from build123d import *

# Parameters (mm, degrees)
F0_W     = 6.35
F0_H     = 28.575
F0_H_2   = 31.75
F0_W_2   = 69.723
F1_DEPTH = 25.4
F2_DEPTH = 6.35
F3_DEPTH = 6.35
F4_DEPTH = 11.176
F7_DEPTH = 6.35


with BuildPart() as f1:
    # F0 (on Top) → F1 (new body)
    with BuildSketch(Plane.XY):
        with Locations((3.175, 14.2875)):
            Rectangle(F0_W, F0_H)
        Polygon((6.35, 28.575), (6.35, 0), (69.596, 0), (69.596, 17.526), (87.122, 17.526), (76.073, 28.575), align=None)
        with BuildLine():
            ThreePointArc((30.988, 8.636), (25.4, 14.224), (30.988, 19.812))
            Line((30.988, 19.812), (54.864, 19.812))
            ThreePointArc((54.864, 19.812), (60.452, 14.224), (54.864, 8.636))
            Line((54.864, 8.636), (30.988, 8.636))
        make_face(mode=Mode.SUBTRACT)
        with Locations((3.175, 44.45)):
            Rectangle(F0_W, F0_H_2)
        Polygon((69.596, 17.526), (69.596, 0), (104.648, 0), (87.122, 17.526), align=None)
        with Locations((41.2115, 44.45)):
            Rectangle(F0_W_2, F0_H_2)
        with Locations((3.175, 74.6125)):
            Rectangle(F0_W, F0_H)
        Polygon((6.35, 88.9), (6.35, 60.325), (76.073, 60.325), (87.122, 71.374), (69.596, 71.374), (69.596, 88.9), align=None)
        with BuildLine():
            Line((54.864, 69.088), (30.988, 69.088))
            ThreePointArc((30.988, 69.088), (25.4, 74.676), (30.988, 80.264))
            Line((30.988, 80.264), (54.864, 80.264))
            ThreePointArc((54.864, 80.264), (60.452, 74.676), (54.864, 69.088))
        make_face(mode=Mode.SUBTRACT)
        Polygon((69.596, 71.374), (87.122, 71.374), (104.648, 88.9), (69.596, 88.9), align=None)
    extrude(amount=-F1_DEPTH)

    # F0 (on Top) → F2 (cut)
    with BuildSketch(Plane.XY):
        Polygon((6.35, 28.575), (6.35, 0), (69.596, 0), (69.596, 17.526), (87.122, 17.526), (76.073, 28.575), align=None)
        with BuildLine():
            ThreePointArc((30.988, 8.636), (25.4, 14.224), (30.988, 19.812))
            Line((30.988, 19.812), (54.864, 19.812))
            ThreePointArc((54.864, 19.812), (60.452, 14.224), (54.864, 8.636))
            Line((54.864, 8.636), (30.988, 8.636))
        make_face(mode=Mode.SUBTRACT)
    extrude(amount=-F2_DEPTH, mode=Mode.SUBTRACT)

    # F0 (on Top) → F3 (cut)
    with BuildSketch(Plane.XY):
        Polygon((6.35, 88.9), (6.35, 60.325), (76.073, 60.325), (87.122, 71.374), (69.596, 71.374), (69.596, 88.9), align=None)
        with BuildLine():
            Line((54.864, 69.088), (30.988, 69.088))
            ThreePointArc((30.988, 69.088), (25.4, 74.676), (30.988, 80.264))
            Line((30.988, 80.264), (54.864, 80.264))
            ThreePointArc((54.864, 80.264), (60.452, 74.676), (54.864, 69.088))
        make_face(mode=Mode.SUBTRACT)
    extrude(amount=-F3_DEPTH, mode=Mode.SUBTRACT)

    # F0 (on Top) → F4 (cut)
    with BuildSketch(Plane.XY):
        with Locations((3.175, 14.2875)):
            Rectangle(F0_W, F0_H)
        with Locations((3.175, 44.45)):
            Rectangle(F0_W, F0_H_2)
        with Locations((3.175, 74.6125)):
            Rectangle(F0_W, F0_H)
    extrude(amount=-F4_DEPTH, mode=Mode.SUBTRACT)

    # F6 (on offset) → F7 (cut)
    with BuildSketch(Plane.XY.offset(-25.4)):
        Polygon((0, 28.575), (0, 0), (69.596, 0), (69.596, 17.526), (87.122, 17.526), (76.073, 28.575), align=None)
        Polygon((0, 88.9), (0, 60.325), (76.073, 60.325), (87.122, 71.374), (69.596, 71.374), (69.596, 88.9), align=None)
    extrude(amount=F7_DEPTH, mode=Mode.SUBTRACT)


solid = f1.part
Source: CAD feature listing. Evaluate the final solid. Frame: model axes, mm. A direction names the side the tool comes from. Round coordinates to 2 decimals unless told otherwise and drop trailing zeros. Loops run counter-clockwise (first coordinate to the right, second up) from the corner with the lowest first, then second, coordinate; pieces in that order, holes last. Notation, with made-up numbers: (32, 45) -> (47, 45) arc R28 cw to (47, 84) -> close; hole circle Ø2 at (86.25, -12.75). An arc over 180 degrees is marked (long way). Answer as a JSON object with one key per item and string values. Group by question number.
Q1. Contact query for flat-ended pins moving along their axis: P1, Ø1, axis at y = 73, z = -11, coming from the +X side; P2, Ø3, axis at x = 39, z = -22, coming from the +Y side (3 decimals); P3, Ø1, axis at y = 48, z = -21.5, coming from the +X side. Output: stop coordinate, or through.
Q2. Section query C-C (x = 68). Output: boundary loops of the cut face in (y, z) (3 decimals), plus the area to 3 significant figures.
Q3. Mould query, pull axis Y, two halves, no side actions, for faces 5 (the flat face through (0, 45, -17)), 6 (the flat face through (65, 88.9, -13)), 7 (the cylindrical face through (25.4, 14.1, -12.6)). Classes: pulls with the +Y half, pulls with the -Y half, needs draft (parallel to the pull), parting line crosses it, or undercut.
Q4. Access query for faces 1 (the flat face through (69.596, 80, -22)), 2 (the flat face through (43, 8.636, -13)), 3 (the flat face through (69.596, 9, -22)), 4 (the flat face through (6.35, 44, -7)). Directions: +Z, -Z, +X, -X, +Y, -Y. A direction counts if a zero-diameter tool reaches every point of the face in a straight line with its end or side. Return the directions, or none.
Q5. Section query D-D (z = -21.5). Output: boundary loops of the cut face in (x, y) (3 decimals), plus the area to 3 significant figures.
Q6. Ray query, line 1 (Y direction, x = 71, z = -3.5) (3 decimals); line 2 (Y direction, x = 6.5, z = -4.25) (3 decimals); line 3 (X direction, y = 33, z = -5.75). Return the intervals inside material, ascending. Write a range as from..to.
Q7. Section query B-B (z = -10). Output: boundary loops of the cut face in (x, y) (3 decimals).
Q8. Section query A-A (x = 51). Output: boundary loops of the cut face in (y, z) (3 decimals), plus the area to 3 significant figures.
Completed:
{
 "1": {"P1": "x = 89.25", "P2": "y = 60.325", "P3": "x = 76.07"},
 "2": {"outline": "(0, -19.05) -> (28.575, -19.05) -> (28.575, -25.4) -> (60.325, -25.4) -> (60.325, -19.05) -> (88.9, -19.05) -> (88.9, -6.35) -> (60.325, -6.35) -> (60.325, 0) -> (28.575, 0) -> (28.575, -6.35) -> (0, -6.35) -> close", "area": "1,530 mm²"},
 "3": {"face 5": "needs draft", "face 6": "pulls with the +Y half", "face 7": "undercut"},
 "4": {"face 1": "-Z, -X, +Y", "face 2": "+Z, -Z", "face 3": "-Z, -X, -Y", "face 4": "+Z, -X, +Y, -Y"},
 "5": {"outline": "(0, 28.575) -> (76.073, 28.575) -> (76.073, 60.325) -> (0, 60.325) -> close; (69.596, 0) -> (104.648, 0) -> (87.122, 17.526) -> (69.596, 17.526) -> close; (69.596, 71.374) -> (87.122, 71.374) -> (104.648, 88.9) -> (69.596, 88.9) -> close", "area": "3,340 mm²"},
 "6": {"line 1": "0..17.526, 28.575..60.325, 71.374..88.9", "line 2": "28.575..60.325", "line 3": "6.35..76.07"},
 "7": {"outline": "(6.35, 0) -> (104.648, 0) -> (76.073, 28.575) -> (76.073, 60.325) -> (104.648, 88.9) -> (6.35, 88.9) -> close; hole (30.988, 8.636) -> (54.864, 8.636) arc R5.588 ccw to (54.864, 19.812) -> (30.988, 19.812) arc R5.588 ccw to start; hole (30.988, 69.088) -> (54.864, 69.088) arc R5.588 ccw to (54.864, 80.264) -> (30.988, 80.264) arc R5.588 ccw to start"},
 "8": {"outline": "(0, -19.05) -> (8.636, -19.05) -> (8.636, -6.35) -> (0, -6.35) -> close; (19.812, -19.05) -> (28.575, -19.05) -> (28.575, -25.4) -> (60.325, -25.4) -> (60.325, -19.05) -> (69.088, -19.05) -> (69.088, -6.35) -> (60.325, -6.35) -> (60.325, 0) -> (28.575, 0) -> (28.575, -6.35) -> (19.812, -6.35) -> close; (80.264, -19.05) -> (88.9, -19.05) -> (88.9, -6.35) -> (80.264, -6.35) -> close", "area": "1,250 mm²"}
}
